Read the model definition and answer for the solid it produces. Units are mm, in the model's axes. Face numbers are marked on the shaded views. A direction names the side the tool comes from. Give positions to 0.01 mm unless a question says otherwise; leave off trailing zeros. Loops run counter-clockwise (first coordinate to the right, second up) from the corner with the lowest first, then second, coordinate; pieces in that order, holes last.
(1) Find section A-A, the plane z = 2.5. Write down the section's boundary in (x, y).
(2) Straight lines are drawn through the part: probe 1 along Y at (x, z) = (1, 7.75); probe 2 along Y at (x, z) = (-0.25, 3.25); probe 3 along X at (y, z) = (63, 3.75). For each, find the intervals that lie inside material, in ascending order.
(3) Which of the six approach directions +Z, -Z, +X, -X, +Y, -Y give full straight-line access (tool end or side, diameter ignored) to the marked faces 1, 2 and 3?
(4) Find section B-B, the plane y = 87. Write down the section's boundary in (x, z), then the cut area to 3 significant figures.
(5) Find section C-C, the plane y = 21. Write down the section's boundary in (x, z).
(6) Each of these flat-tipped pins is pushed along its axis until it touches: P1, Ø3, axis at y = 46.5, z = 9, coming from the -X side; P2, Ø1, axis at x = -2.5, z = 7.5, coming from the +Y side; P3, Ø4, axis at x = 2.5, y = 40.5, coming from the +Z side. Where does it stop, or does it pass through?
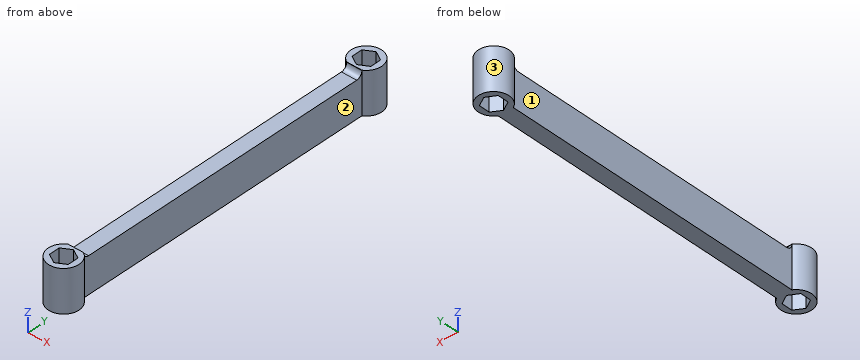
```python
from build123d import *

# Parameters (mm, degrees)
PAD_DEPTH       = 11
POCKET_DEPTH    = 11.001
SKETCH002_W     = 80.071796
SKETCH002_H     = 1.6
POCKET001_DEPTH = 6.001
FILLET_R        = 1.5
FILLET001_R     = 1.5


with BuildPart() as part:
    # Sketch → Pad (new body)
    with BuildSketch(Plane.XY):
        with BuildLine():
            ThreePointArc((-2, 3.464102), (0, -4), (2, 3.464102))
            Line((2, 83.535898), (2, 3.464102))
            ThreePointArc((2, 83.535898), (0, 91), (-2, 83.535898))
            Line((-2, 83.535898), (-2, 3.464102))
        make_face()
    extrude(amount=PAD_DEPTH)

    # Sketch001 (on Face6 of Pad) → Pocket (cut, through all)
    with BuildSketch(Plane.XY.offset(11)):
        Polygon((2.45, 85.585492), (2.45, 88.414508), (0, 89.829016), (-2.45, 88.414508), (-2.45, 85.585492), (0, 84.170984), align=None)
        Polygon((2.45, -1.414508), (2.45, 1.414508), (0, 2.829016), (-2.45, 1.414508), (-2.45, -1.414508), (0, -2.829016), align=None)
    extrude(amount=-POCKET_DEPTH, mode=Mode.SUBTRACT)

    # Sketch002 (on Face2 of Pocket) → Pocket001 (cut, through all)
    with BuildSketch(Plane.YZ.offset(2)):
        with Locations((43.5, 10.2)):
            Rectangle(SKETCH002_W, SKETCH002_H)
    extrude(amount=-POCKET001_DEPTH, mode=Mode.SUBTRACT)

    # Fillet
    fillet_edges = [part.edges().sort_by_distance(p)[0] for p in [
        (0, 83.535898, 9.4),
    ]]
    fillet(fillet_edges, radius=FILLET_R)

    # Fillet001
    fillet001_edges = [part.edges().sort_by_distance(p)[0] for p in [
        (0, 3.464102, 9.4),
    ]]
    fillet(fillet001_edges, radius=FILLET001_R)


solid = part.part
```
Entries:
1. outline: (-2, 3.46) arc R4 ccw (long way) to (2, 3.46) - (2, 83.54) arc R4 ccw (long way) to (-2, 83.54) - close; hole (-2.45, -1.41) - (0, -2.83) - (2.45, -1.41) - (2.45, 1.41) - (0, 2.83) - (-2.45, 1.41) - close; hole (-2.45, 85.59) - (0, 84.17) - (2.45, 85.59) - (2.45, 88.41) - (0, 89.83) - (-2.45, 88.41) - close
2. probe 1: y = -3.87 to -2.25, 2.25 to 84.75, 89.25 to 90.87
2. probe 2: y = -3.99 to -2.68, 2.68 to 84.32, 89.68 to 90.99
2. probe 3: x = -2 to 2
3. face 1: +Z, -Z, -X
3. face 2: +Z, -Z, +X
3. face 3: +Z, -Z
4. outline: (-4, 0) - (-2.45, 0) - (-2.45, 11) - (-4, 11) - close; (2.45, 0) - (4, 0) - (4, 11) - (2.45, 11) - close
4. area: 34.1 mm2
5. outline: (-2, 0) - (2, 0) - (2, 9.4) - (-2, 9.4) - close
6. P1: stops at x = -2
6. P2: stops at y = 90.46
6. P3: stops at z = 9.4
